Can you work these out from the drawing? Everything is in mm from the part's minimum corner. A direction names the side the tool comes from. Give positions to 0.01 mm unless a question says otherwise; leave off trailing zeros. Write each loop counter-clockwise with the first axis right and the second up, starting at its lowest first coordinate (ties: lowest second). Pieces come first, ordered by that corner, then holes. Notation, with made-up numbers: M -15.5,66.25 L 13.5,66.25 A19 cw 13.5,82.25 Z; hole C 67.5,38.25 d7. An arc over 180 degrees is marked long. One line per item, written item: value.
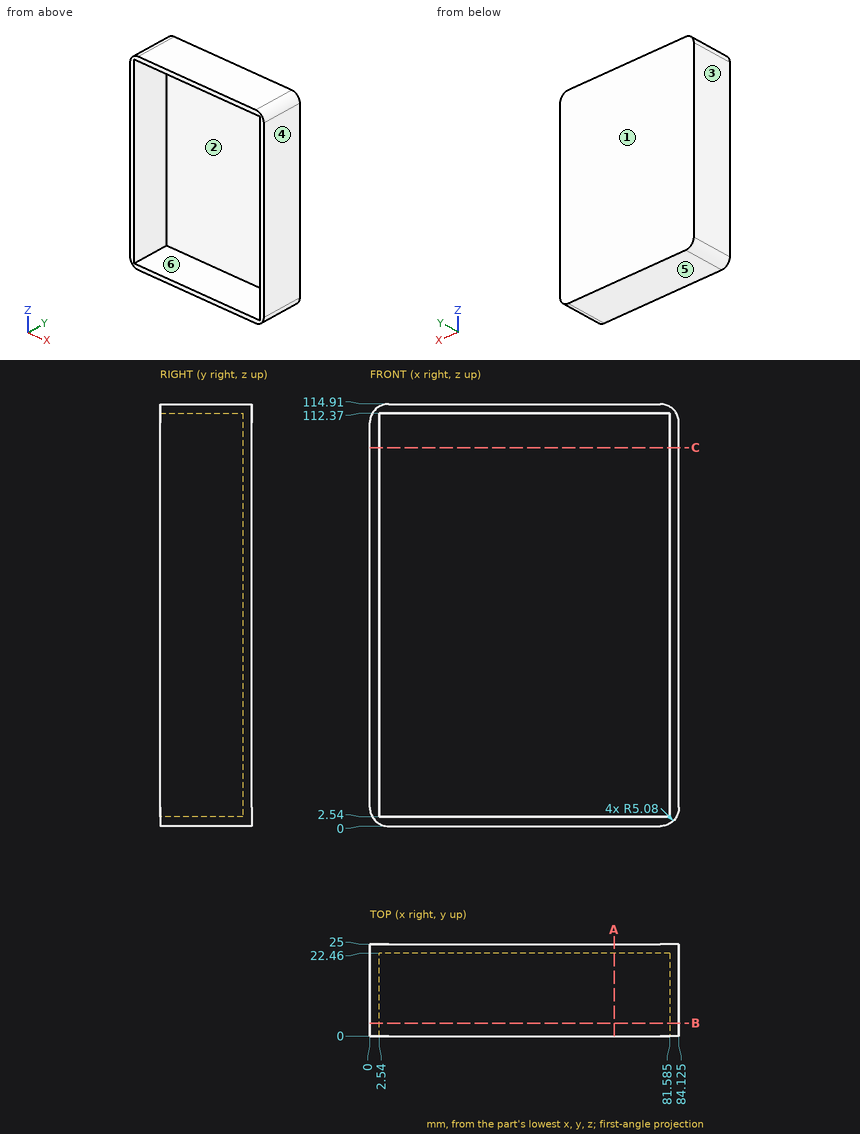
1) We'd pull the mould along X, two halves only. Please class the marked faces 1, 2, 3 and 4: pulls with the +X half, pulls with the -X half, needs draft (parallel to the pull), parting line crosses it, or undercut.
Outcome:
face 1: needs draft
face 2: undercut
face 3: pulls with the -X half
face 4: pulls with the +X half
2) On a 3-axis mill with a long thin cutter (end or side, diameter ignored), from which of +Z, -Z, +X, -X, +Y, -Y can I reach the whole of each face in a straight line? I mean the marked faces 5 and 6. Say none if no direction works.
Outcome:
face 5: -Z, +X, -X, +Y, -Y
face 6: -Y
3) If we section it at B-B, the plane y = 3.5: Write out the boundary of the cut face in (x, z) (1 decimal).
Outcome:
outline: M 0,5.1 A5.1 ccw 5.1,0 L 79,0 A5.1 ccw 84.1,5.1 L 84.1,109.8 A5.1 ccw 79,114.9 L 5.1,114.9 A5.1 ccw 0,109.8 Z; hole M 2.5,2.5 L 81.6,2.5 L 81.6,112.4 L 2.5,112.4 Z
4) If we section it at A-A, the plane x = 66.5: Write out the boundary of the cut face in (y, z), then the cut area to 3 significant figures.
Outcome:
outline: M 0,0 L 25,0 L 25,114.91 L 0,114.91 L 0,112.37 L 22.46,112.37 L 22.46,2.54 L 0,2.54 Z
area: 406 mm^2
5) Please list where these lines run through material, in increasing order: L1, parallel to Z at x = 66, y = 11.75; L2, parallel to X at y = 2.75, z = 9 (1 decimal); L3, parallel to Y at x = 34, z = 101.5. Write a range as from..to.
Outcome:
L1: z = 0..2.54, 112.37..114.91
L2: x = 0..2.5, 81.6..84.1
L3: y = 22.46..25
6) If we section it at C-C, the plane z = 103: Write out the boundary of the cut face in (x, y) (1 decimal).
Outcome:
outline: M 0,0 L 2.5,0 L 2.5,22.5 L 81.6,22.5 L 81.6,0 L 84.1,0 L 84.1,25 L 0,25 Z
7) I'm going to push a flat-ended pin straight in: pin 1 (23.5 mm diameter, centred on x = 53.5, z = 79, fed in from -Y). Where does the tip first touch, or does it pass through?
Outcome:
pin 1: stops at y = 22.46
